For this review, use the dimensioned drawing (mm, ordinates from the lowest corner) and the shaded views. A direction names the side the tool comes from. Round coordinates to 2 decimals unless told otherwise and drop trailing zeros. Write each loop counter-clockwise with the first axis right and the second up, starting at its lowest first coordinate (ties: lowest second). Pieces come first, ordered by that corner, then holes. Notation, with made-up numbers: (45.5, -21.5) - (57.5, -21.5) arc R14 ccw to (57.5, -3.5) - close; hole circle Ø5 at (23, -26). An arc over 180 degrees is marked (long way). Write each question's results on one line, items separated by ' | '.
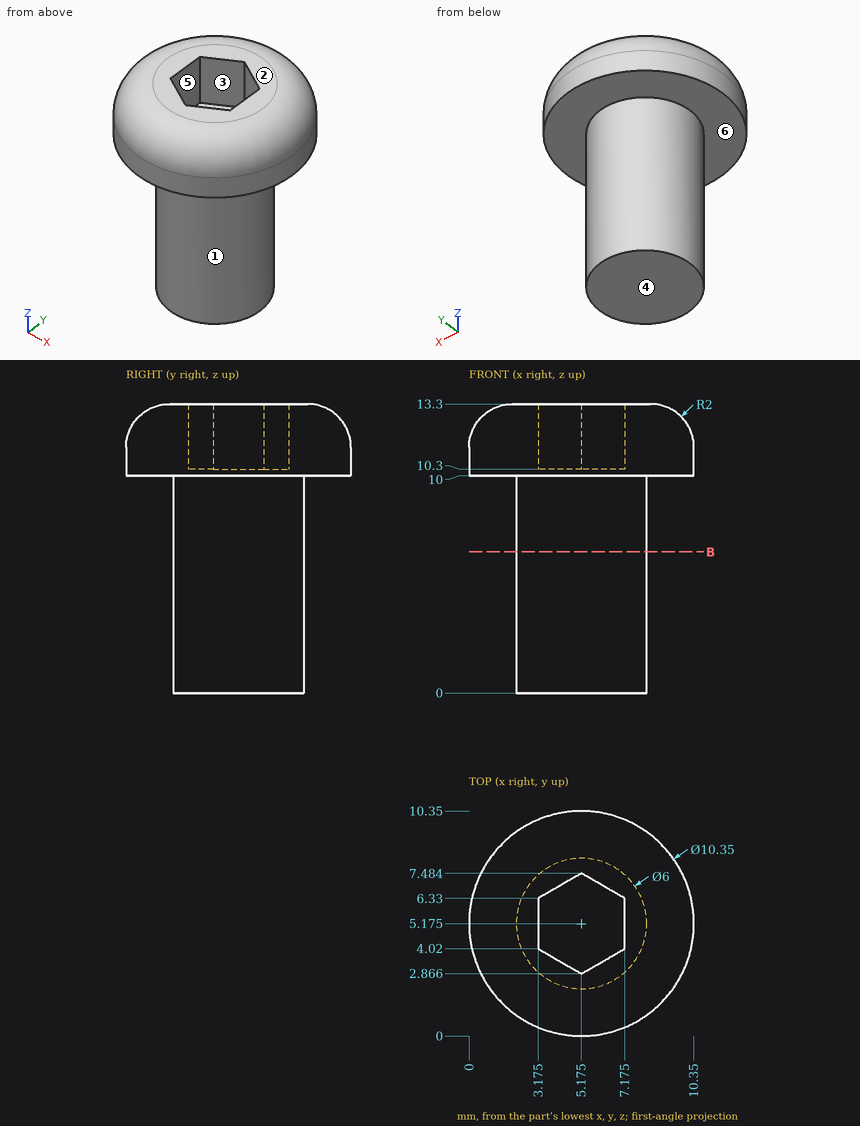
Q1. For probe 1 along Z at (x, y) = (3.25, 6.25); probe 2 along X at (y, z) = (5.5, 12.5) (1 decimal); probe 3 along X at (y, z) = (5.25, 9.5), list the stretches that pass through material, from the lowest coordinate up.
Evaluation:
probe 1: z = 0 to 10.3 | probe 2: x = 0.4 to 3.2, 7.2 to 9.9 | probe 3: x = 2.18 to 8.17
Q2. Insertion check: P1, Ø1, axis at x = 8.5, z = 10, coming from the -Y side; P2, Ø1.2, axis at y = 5.5, z = 12.5, coming from the +X side; P3, Ø1.2, axis at y = 5, z = 12.5, coming from the -X side (1 decimal). Each pin has a flat end and moves straight along its axis. Give the tip position at first contact, or say it passes through.
Evaluation:
P1: stops at y = 0.84 | P2: stops at x = 10.25 | P3: stops at x = 0.1
Q3. Tool access review of the marked faces 4, 5 and 6: name each direction out of +Z, -Z, +X, -X, +Y, -Y from which nothing blocks a thin tool from reaching the whole face with its end or side.
Evaluation:
face 4: -Z, +X, -X, +Y, -Y | face 5: +Z | face 6: -Z
Q4. The part is to be moulded in two halves that separate along Y. For the marked faces 1, 2 and 3, say which applies: released by +Y, released by -Y, zero draft, split by the parting line, or undercut.
Evaluation:
face 1: split by the parting line | face 2: zero draft | face 3: undercut
Q5. We need section B-B (z = 6.5). State the section outline as (x, y) points (1 decimal), plus the area to 3 significant figures.
Evaluation:
outline: circle Ø6 at (5.2, 5.2) | area: 28.3 mm^2
